```python
from build123d import *

# Parameters (mm, degrees)
SKETCH1_W           = 33.45
SKETCH1_H           = 10.5
BOSS_EXTRUDE1_DEPTH = 3
BOSS_EXTRUDE2_DEPTH = 10.5
CUT_EXTRUDE1_REACH  = 40.598
SKETCH3_R           = 1.5825


with BuildPart() as part:
    # Sketch1 → Boss-Extrude1 (new body)
    with BuildSketch(Plane.XY):
        with Locations((16.725, 5.25)):
            Rectangle(SKETCH1_W, SKETCH1_H)
    extrude(amount=BOSS_EXTRUDE1_DEPTH)

    # Sketch2 → Boss-Extrude2 (add)
    with BuildSketch(Plane.XZ):
        with BuildLine():
            Line((33.45, 3), (33.45, 10))
            ThreePointArc((33.45, 10), (26.127788274, 15.197537565), (17.167255211, 15.778939776))
            ThreePointArc((17.167255211, 15.778939776), (13.513268499, 14.036363917), (10.822706511, 11.011621661))
            ThreePointArc((10.822706511, 11.011621661), (6.874462981, 8.368470255), (2.551142404, 10.339199946))
            Line((2.551142404, 10.339199946), (2.551142404, 8.639199946))
            ThreePointArc((2.551142404, 8.639199946), (4.602955754, 7.079155178), (7.145952658, 6.658626408))
            ThreePointArc((7.145952658, 6.658626408), (10.559689681, 8.1799455), (12.998874454, 11.011621661))
            ThreePointArc((12.998874454, 11.011621661), (14.440986225, 12.472256001), (16.259204718, 13.424737261))
            ThreePointArc((16.259204718, 13.424737261), (18.189418616, 13.879021589), (20.168677104, 14))
            ThreePointArc((20.168677104, 14), (25.739491976, 13.10563656), (30.45, 10))
            Line((30.45, 10), (30.45, 3))
            Line((30.45, 3), (33.45, 3))
        make_face()
    extrude(amount=-BOSS_EXTRUDE2_DEPTH)

    # Sketch3 → Cut-Extrude1 (cut, up to next)
    with BuildSketch(Plane(origin=(0, 0, 0), x_dir=(-1, 0, 0), z_dir=(0, 0, -1)), mode=Mode.PRIVATE) as cut_extrude1_sk1:
        with Locations((-9, 5.25)):
            Circle(SKETCH3_R)
    cut_extrude1_tool1 = extrude(cut_extrude1_sk1.sketch, amount=-CUT_EXTRUDE1_REACH, mode=Mode.PRIVATE) & part.part
    add(cut_extrude1_tool1.solids().sort_by_distance((9, 5.25, 0))[0], mode=Mode.SUBTRACT)


solid = part.part
```
For this review, take the finished solid that the model builds, in its own axes (mm). A direction names the side the tool comes from. Round coordinates to 2 decimals unless told otherwise and drop trailing zeros. Order: outer loops, then holes, each group sorted by start corner. A loop starts at its lowest first (then second) coordinate and runs counter-clockwise, first axis right, second up. Notation, with made-up numbers: (-30, -37.75) -> (5, -37.75) arc R6 cw to (5, -27.75) -> close; hole circle Ø8 at (-14, 80). An arc over 180 degrees is marked (long way). Use a Markdown table: item, result.
Item 1: Take a section at C-C (z = 9.25). State the section outline as (x, y) points.
Resolved:
| item | result |
|---|---|
| outline | (2.55, 0) -> (3.66, 0) -> (3.66, 10.5) -> (2.55, 10.5) -> close; (9.3, 0) -> (11.75, 0) -> (11.75, 10.5) -> (9.3, 10.5) -> close; (30.45, 0) -> (33.45, 0) -> (33.45, 10.5) -> (30.45, 10.5) -> close |
Item 2: Draft analysis for pull direction X (two halves, no side actions). For faces 4 (the cylindrical face through (13.6, 5.2, 14.1)), 5 (the cylindrical face through (10.52, 5.18, 8.15)), 6 (the cylindrical face through (14.418, 5.176, 12.455)), 7 (the flat face through (20.2, 10.5, 2.8)), state which applies: +X half, -X half, draft (parallel to the pull), parting line (faces both ways), or undercut.
Resolved:
| item | result |
|---|---|
| face 4 | -X half |
| face 5 | undercut |
| face 6 | undercut |
| face 7 | draft |
Item 3: Take a section at B-B (x = 9). State the section outline as (y, z) points, plus the area to 3 significant figures.
Resolved:
| item | result |
|---|---|
| outline | (0, 0) -> (3.67, 0) -> (3.67, 3) -> (0, 3) -> close; (0, 7.26) -> (10.5, 7.26) -> (10.5, 9.05) -> (0, 9.05) -> close; (6.83, 0) -> (10.5, 0) -> (10.5, 3) -> (6.83, 3) -> close |
| area | 40.9 mm² |
Item 4: Take a section at A-A (y = 5.25). State the section outline as (x, z) points, plus the area to 3 significant figures.
Resolved:
| item | result |
|---|---|
| outline | (0, 0) -> (7.42, 0) -> (7.42, 3) -> (0, 3) -> close; (2.55, 8.64) arc R5.35 ccw to (7.15, 6.66) arc R8.55 ccw to (13, 11.01) arc R6.66 cw to (16.26, 13.42) arc R11.67 cw to (20.17, 14) arc R13.42 cw to (30.45, 10) -> (30.45, 3) -> (10.58, 3) -> (10.58, 0) -> (33.45, 0) -> (33.45, 10) arc R16.46 ccw to (17.17, 15.78) arc R10.22 ccw to (10.82, 11.01) arc R4.88 cw to (2.55, 10.34) -> close |
| area | 177 mm² |
Item 5: Take a section at D-D (y = 9.5). State the section outline as (x, z) points.
Resolved:
| item | result |
|---|---|
| outline | (0, 0) -> (33.45, 0) -> (33.45, 10) arc R16.46 ccw to (17.17, 15.78) arc R10.22 ccw to (10.82, 11.01) arc R4.88 cw to (2.55, 10.34) -> (2.55, 8.64) arc R5.35 ccw to (7.15, 6.66) arc R8.55 ccw to (13, 11.01) arc R6.66 cw to (16.26, 13.42) arc R11.67 cw to (20.17, 14) arc R13.42 cw to (30.45, 10) -> (30.45, 3) -> (0, 3) -> close |
Item 6: Machinability: for faces 1 (the flat face through (2.551, 5, 10)), 2 (the flat face through (15, 5, 3)), 3 (the flat face through (30.45, 5, 7)), which of the approach directions +Z, -Z, +X, -X, +Y, -Y give a long, thin tool a straight path to every point of the face, cutting with its end or side? Answer none if there is none.
Resolved:
| item | result |
|---|---|
| face 1 | +Z, -X, +Y, -Y |
| face 2 | -X, +Y, -Y |
| face 3 | +Y, -Y |
Item 7: For line 1 along X through (y, z) = (4.5, 8.75); line 2 along Y through (x, z) = (9, 1.8); line 3 along X through (y, z) = (8.5, 6.5), list the stretches that pass through material, from the lowest coordinate up. Write a range as [from, to].
Resolved:
| item | result |
|---|---|
| line 1 | x = [2.55, 4.55], [8.41, 11.25], [30.45, 33.45] |
| line 2 | y = [0, 3.67], [6.83, 10.5] |
| line 3 | x = [30.45, 33.45] |
Item 8: For pin 1 (3 mm diameter, centred on y = 7.5, z = 7, fed in from -X); pin 2 (3.5 mm diameter, centred on y = 4.5, z = 7, fed in from -X); pin 3 (1 mm diameter, centred on x = 4.5, z = 5, fed in from -Y); pin 4 (4 mm diameter, centred on x = 14.5, y = 5, fed in from +Z), all flat-tipped, find the tip position at first contact; note any pin that passes through.
Resolved:
| item | result |
|---|---|
| pin 1 | stops at x = 2.67 |
| pin 2 | stops at x = 2.55 |
| pin 3 | passes through |
| pin 4 | stops at z = 15.59 |
